from build123d import *

# Parameters (mm, degrees)
EXTRUDE_1_DEPTH     = 10
SKETCH_2_R          = 1.5
CUT_EXTRUDE_1_DEPTH = 10
SKETCH_3_R          = 1.5
CUT_EXTRUDE_2_DEPTH = 10
SKETCH_4_R          = 1.5
CUT_EXTRUDE_3_DEPTH = 10
SKETCH_5_W          = 35
SKETCH_5_H          = 24
CUT_EXTRUDE_4_DEPTH = 6
SKETCH_6_R          = 1.5
CUT_EXTRUDE_5_DEPTH = 241.956427596


with BuildPart() as part:
    # 草图1 → 凸台-拉伸1 (new body)
    with BuildSketch(Plane.XY):
        with BuildLine():
            Line((118, 210), (-118, 210))
            Line((-118, 210), (-118, -210))
            Line((-118, -210), (118, -210))
            Line((118, -210), (118, -50.5))
            Line((118, -50.5), (40.5, -50.5))
            Line((40.5, -50.5), (40.5, -9.334147293))
            ThreePointArc((40.5, -9.334147293), (24.099506706, 0), (40.5, 9.334147293))
            Line((40.5, 9.334147293), (40.5, 50.5))
            Line((40.5, 50.5), (118, 50.5))
            Line((118, 50.5), (118, 210))
        make_face()
    extrude(amount=EXTRUDE_1_DEPTH)

    # 草图2 → 切除-拉伸1 (cut)
    with BuildSketch(Plane.XY.offset(10)):
        with Locations((-98, 165)):
            Circle(SKETCH_2_R)
        with Locations((-73, 190)):
            Circle(SKETCH_2_R)
        with Locations((-98, 190)):
            Circle(SKETCH_2_R)
    cut_extrude_1 = extrude(amount=-CUT_EXTRUDE_1_DEPTH, mode=Mode.SUBTRACT)

    # 草图3 → 切除-拉伸2 (cut)
    with BuildSketch(Plane.XY.offset(10)):
        with Locations((37.5, -15.672792958)):
            Circle(SKETCH_3_R)
        with Locations((112.73, -53.5)):
            Circle(SKETCH_3_R)
        with Locations((112.73, -59.5)):
            Circle(SKETCH_3_R)
        with Locations((87.23, -53.5)):
            Circle(SKETCH_3_R)
        with Locations((87.23, -59.5)):
            Circle(SKETCH_3_R)
        with Locations((77.23, -53.5)):
            Circle(SKETCH_3_R)
        with Locations((61.23, -53.5)):
            Circle(SKETCH_3_R)
        with Locations((37.5, -53.5)):
            Circle(SKETCH_3_R)
        with Locations((37.5, -43.5)):
            Circle(SKETCH_3_R)
    cut_extrude_2 = extrude(amount=-CUT_EXTRUDE_2_DEPTH, mode=Mode.SUBTRACT)

    # 镜向1: 切除-拉伸2 across plane
    add(cut_extrude_2.mirror(Plane.ZX), mode=Mode.SUBTRACT)

    # 镜向2: 切除-拉伸1 across plane
    add(cut_extrude_1.mirror(Plane.ZX), mode=Mode.SUBTRACT)

    # 草图4 → 切除-拉伸3 (cut)
    with BuildSketch(Plane.XY.offset(10)):
        with Locations((32, 180)):
            Circle(SKETCH_4_R)
        with Locations((47, 180)):
            Circle(SKETCH_4_R)
    cut_extrude_3 = extrude(amount=-CUT_EXTRUDE_3_DEPTH, mode=Mode.SUBTRACT)

    # 镜向3: 切除-拉伸3 across plane
    add(cut_extrude_3.mirror(Plane.ZX), mode=Mode.SUBTRACT)

    # 草图5 → 切除-拉伸4 (cut)
    with BuildSketch(Plane.XY.offset(10)):
        with Locations((100.5, -188)):
            Rectangle(SKETCH_5_W, SKETCH_5_H)
    cut_extrude_4 = extrude(amount=-CUT_EXTRUDE_4_DEPTH, mode=Mode.SUBTRACT)

    # 草图6 → 切除-拉伸5 (cut, through all)
    with BuildSketch(Plane.XY.offset(4)):
        with Locations((111.75, -179)):
            Circle(SKETCH_6_R)
        with Locations((111.75, -197)):
            Circle(SKETCH_6_R)
    cut_extrude_5 = extrude(amount=-CUT_EXTRUDE_5_DEPTH, mode=Mode.SUBTRACT)

    # 镜向4: 切除-拉伸4, 切除-拉伸5 across plane
    add(cut_extrude_4.mirror(Plane.ZX), mode=Mode.SUBTRACT)
    add(cut_extrude_5.mirror(Plane.ZX), mode=Mode.SUBTRACT)


solid = part.part
Can you work these out from the model? Positions are in its coordinate system, mm. A direction names the side the tool comes from. Give positions to 0.01 mm unless a question says otherwise; leave off trailing zeros. Loops run counter-clockwise (first coordinate to the right, second up) from the corner with the lowest first, then second, coordinate; pieces in that order, holes last. Notation, with made-up numbers: (11.25, 0) -> (68.25, 0) arc R25 ccw to (68.25, 35) -> close; hole circle Ø9 at (10.25, 11). An arc over 180 degrees is marked (long way). Use one line per item in the form item = value.
1) I need wall thicknesses on line 1 along Y through (x, z) = (-73, 7.75); line 2 along Y through (x, z) = (-98, 4); line 3 along Y through (x, z) = (53, 2.75). Which ranges of each line are inside material? Lowest first, please.
Answers:
line_1 = -210 to -191.5, -188.5 to 188.5, 191.5 to 210
line_2 = -210 to -191.5, -188.5 to -166.5, -163.5 to 163.5, 166.5 to 188.5, 191.5 to 210
line_3 = -210 to -50.5, 50.5 to 210
2) For faces 1 (the face through (-2, 3, 0)), 2 (the face through (100, 188, 4)), 3 (the face through (80, -50.5, 5)), which set-ups out of +Z, -Z, +X, -X, +Y, -Y let a thin tool reach every point of the face, with its end or its side?
Answers:
face_1 = -Z, +X, -X, +Y, -Y
face_2 = +Z, +X
face_3 = +Z, -Z, +X
3) We'd pull the mould along X, two halves only. Please class faces 4 (the face through (100, -188, 4)), 5 (the face through (24.104, -0.32, 4.93)), 6 (the face through (40.5, 30, 5)), 7 (the face through (-118, 3, 5)): released by +X, released by -X, zero draft, split by the parting line, or undercut.
Answers:
face_4 = zero draft
face_5 = undercut
face_6 = released by +X
face_7 = released by -X
4) If we section it at B-B (z = 7.5): Count the separate pieces of the cut face and the enclosed holes in it, plus the area to 3 significant figures.
Answers:
separate_pieces = 1
enclosed_holes = 28
area = 89,100 mm²
5) Will these pins go through, and if not, where does the flat tip stop? pin 1 (7 mm diameter, centred on x = 106.5, y = 184.5, fed in from +Z); pin 2 (2.5 mm diameter, centred on x = 112.73, y = -53.5, fed in from +Z).
Answers:
pin_1 = 4
pin_2 = through
6) If we section it at A-A (x = 54): Please give me the cut outline in (y, z), plus the area to 3 significant figures.
Answers:
outline = (-210, 0) -> (-50.5, 0) -> (-50.5, 10) -> (-210, 10) -> close; (50.5, 0) -> (210, 0) -> (210, 10) -> (50.5, 10) -> close
area = 3,190 mm²
